from build123d import *

# Parameters (mm, degrees)
SKETCH1_R           = 7.9375
SKETCH1_R_2         = 2.413
BOSS_EXTRUDE1_DEPTH = 7.62
SKETCH2_R           = 7.9375
SKETCH2_R_2         = 3.81
BOSS_EXTRUDE2_DEPTH = 2.54
SKETCH3_W           = 154.94
SKETCH3_H           = 11.43
BOSS_EXTRUDE3_DEPTH = 15.24
FILLET1_R           = 5.08
BOSS_EXTRUDE4_DEPTH = 7.62
SKETCH5_R           = 2.286
CUT_EXTRUDE1_DEPTH  = 128
CUT_EXTRUDE2_DEPTH  = 6.35


with BuildPart() as part:
    # Sketch1 → Boss-Extrude1 (new body)
    with BuildSketch(Plane(origin=(0, 0, 0), x_dir=(0, 0, -1), z_dir=(1, 0, 0))):
        with BuildLine():
            Line((0, 0), (127, 0))
            Line((127, 0), (100.900837488, 6.993249518))
            ThreePointArc((100.900837488, 6.993249518), (97.889599245, 8.807630529), (96.305117976, 11.94593474))
            ThreePointArc((96.305117976, 11.94593474), (85.15869513, 22.438273755), (71.738889517, 15.073442623))
            ThreePointArc((71.738889517, 15.073442623), (69.395749913, 12.417671245), (65.994583888, 11.43))
            Line((65.994583888, 11.43), (0, 11.43))
            Line((0, 11.43), (-63.5, 11.43))
            Line((-63.5, 11.43), (-63.5, 127))
            Line((-63.5, 127), (-88.9, 127))
            Line((-88.9, 127), (-88.9, 0))
            Line((-88.9, 0), (0, 0))
        make_face()
        with Locations((83.514716058, 9.525)):
            Circle(SKETCH1_R, mode=Mode.SUBTRACT)
        with Locations((-76.2, 114.3)):
            Circle(SKETCH1_R_2, mode=Mode.SUBTRACT)
        with Locations((-76.2, 88.9)):
            Circle(SKETCH1_R_2, mode=Mode.SUBTRACT)
        with Locations((-76.2, 101.6)):
            Circle(SKETCH1_R_2, mode=Mode.SUBTRACT)
        with Locations((-76.2, 76.2)):
            Circle(SKETCH1_R_2, mode=Mode.SUBTRACT)
    extrude(amount=BOSS_EXTRUDE1_DEPTH)

    # Sketch2 → Boss-Extrude2 (add)
    with BuildSketch(Plane(origin=(7.62, 0, 0), x_dir=(0, 0, -1), z_dir=(1, 0, 0))):
        with Locations((83.514716058, 9.525)):
            Circle(SKETCH2_R)
        with Locations((83.514716058, 9.525)):
            Circle(SKETCH2_R_2, mode=Mode.SUBTRACT)
    extrude(amount=-BOSS_EXTRUDE2_DEPTH)

    # Sketch3 → Boss-Extrude3 (add)
    with BuildSketch(Plane.ZY):
        with Locations((11.43, 5.715)):
            Rectangle(SKETCH3_W, SKETCH3_H)
    extrude(amount=BOSS_EXTRUDE3_DEPTH)

    # Fillet1
    fillet1_edges = [part.edges().sort_by_distance(p)[0] for p in [
        (0, 5.715, -66.04),
    ]]
    fillet(fillet1_edges, radius=FILLET1_R)

    # Sketch4 → Boss-Extrude4 (add)
    with BuildSketch(Plane(origin=(7.62, 0, 0), x_dir=(0, 0, -1), z_dir=(1, 0, 0))):
        Polygon((-63.5, 54.790512242), (-20.139487758, 11.43), (-38.1, 11.43), (-63.5, 36.83), align=None)
    extrude(amount=-BOSS_EXTRUDE4_DEPTH)

    # Sketch5 → Cut-Extrude1 (cut, through all)
    with BuildSketch(Plane.XZ):
        with Locations((-3.81, -50.8)):
            Circle(SKETCH5_R)
        with Locations((-3.81, 0)):
            Circle(SKETCH5_R)
    extrude(amount=-CUT_EXTRUDE1_DEPTH, mode=Mode.SUBTRACT)

    # Sketch6 → Cut-Extrude2 (cut)
    with BuildSketch(Plane.XZ):
        Polygon((1.61593783, -50.8), (-1.097031085, -46.101), (-6.522968915, -46.101), (-9.23593783, -50.8), (-6.522968915, -55.499), (-1.097031085, -55.499), align=None)
        Polygon((-1.097031085, -4.699), (1.61593783, 0), (-1.097031085, 4.699), (-6.522968915, 4.699), (-9.23593783, 0), (-6.522968915, -4.699), align=None)
    extrude(amount=-CUT_EXTRUDE2_DEPTH, mode=Mode.SUBTRACT)


solid = part.part
The listing builds one solid part. Answer for the finished solid, in the listing's coordinates (mm). A direction names the side the tool comes from. Coordinates: 2 decimals unless noted, no trailing zeros. Order: outer loops, then holes, each group sorted by start corner. A loop starts at its lowest first (then second) coordinate and runs counter-clockwise, first axis right, second up. Notation, with made-up numbers: (66, 8.5) -> (116, 8.5) arc R22 ccw to (116, 19.5) -> close; hole circle Ø2 at (64.5, 36.25). An arc over 180 degrees is marked (long way). Answer in a Markdown table with one row per item. Add a question column.
Item 1: Which of the six approach directions +Z, -Z, +X, -X, +Y, -Y give full straight-line access (tool end or side, diameter ignored) to faces 4 (the face through (0, 3, -48)), 5 (the face through (5.08, 13.2, -85.2)), 6 (the face through (4, 24, 63.5)), 7 (the face through (-10, 6, -66.04))?
Item 2: Find section B-B (z = 76.2). Write down the section's boundary in (x, y).
Item 3: Find section C-C (z = 46). Write down the section's boundary in (x, y), then the cut area to 3 significant figures.
Item 4: Find the intervals of material crossed by L1, parallel to Y at x = 3.5, z = 76.2; L2, parallel to X at y = 79.5, z = 67.5; L3, parallel to Y at x = 3.5, z = -33, in increasing order. Write a range as from..to.
Item 5: Find section D-D (y = 59.5). Write down the section's boundary in (x, z), then the cut area to 3 significant figures.
Item 6: Determine the mould class of faces 1 (the face through (3.86, 33.41, 42.12)), 2 (the face through (3.757, 103.635, 74.903)), 3 (the face through (-7.898, 3.131, -2.317)) for opening direction Y: +Y half, -Y half, draft (parallel to the pull), parting line (faces both ways), or undercut.
Item 7: Each of these flat-tipped pins is pushed along its axis until it touches: P1, Ø6, axis at x = 2.5, y = 91, coming from the -Z side; P2, Ø6.5, axis at y = 88.9, z = 76.2, coming from the -X side; P3, Ø1.5, axis at x = 1.5, z = -20, coming from the +Y side; P4, Ø3, axis at y = 76.2, z = 76.2, coming from the +X side. Where does it stop, or does it pass through?
Item 8: Find section A-A (y = 76.2). Write down the section's boundary in (x, z).
Result set:
| question | item | result |
|---|---|---|
| 1 | face 4 | -Y |
| 1 | face 5 | -X |
| 1 | face 6 | +X, -X |
| 1 | face 7 | -Z, -X, +Y, -Y |
| 2 | outline | (-15.24, 0) -> (7.62, 0) -> (7.62, 73.79) -> (0, 73.79) -> (0, 11.43) -> (-15.24, 11.43) -> close; (0, 78.61) -> (7.62, 78.61) -> (7.62, 86.49) -> (0, 86.49) -> close; (0, 91.31) -> (7.62, 91.31) -> (7.62, 99.19) -> (0, 99.19) -> close; (0, 104.01) -> (7.62, 104.01) -> (7.62, 111.89) -> (0, 111.89) -> close; (0, 116.71) -> (7.62, 116.71) -> (7.62, 127) -> (0, 127) -> close |
| 3 | outline | (-15.24, 0) -> (7.62, 0) -> (7.62, 11.43) -> (-15.24, 11.43) -> close; (0, 19.33) -> (7.62, 19.33) -> (7.62, 37.29) -> (0, 37.29) -> close |
| 3 | area | 398 mm² |
| 4 | L1 | y = 0..73.79, 78.61..86.49, 91.31..99.19, 104.01..111.89, 116.71..127 |
| 4 | L2 | x = 0..7.62 |
| 4 | L3 | y = 0..11.43 |
| 5 | outline | (0, 63.5) -> (7.62, 63.5) -> (7.62, 88.9) -> (0, 88.9) -> close |
| 5 | area | 194 mm² |
| 6 | face 1 | +Y half |
| 6 | face 2 | undercut |
| 6 | face 3 | draft |
| 7 | P1 | stops at z = 63.5 |
| 7 | P2 | stops at x = 0 |
| 7 | P3 | stops at y = 11.43 |
| 7 | P4 | passes through |
| 8 | outline | (0, 63.5) -> (7.62, 63.5) -> (7.62, 73.79) -> (0, 73.79) -> close; (0, 78.61) -> (7.62, 78.61) -> (7.62, 88.9) -> (0, 88.9) -> close |
